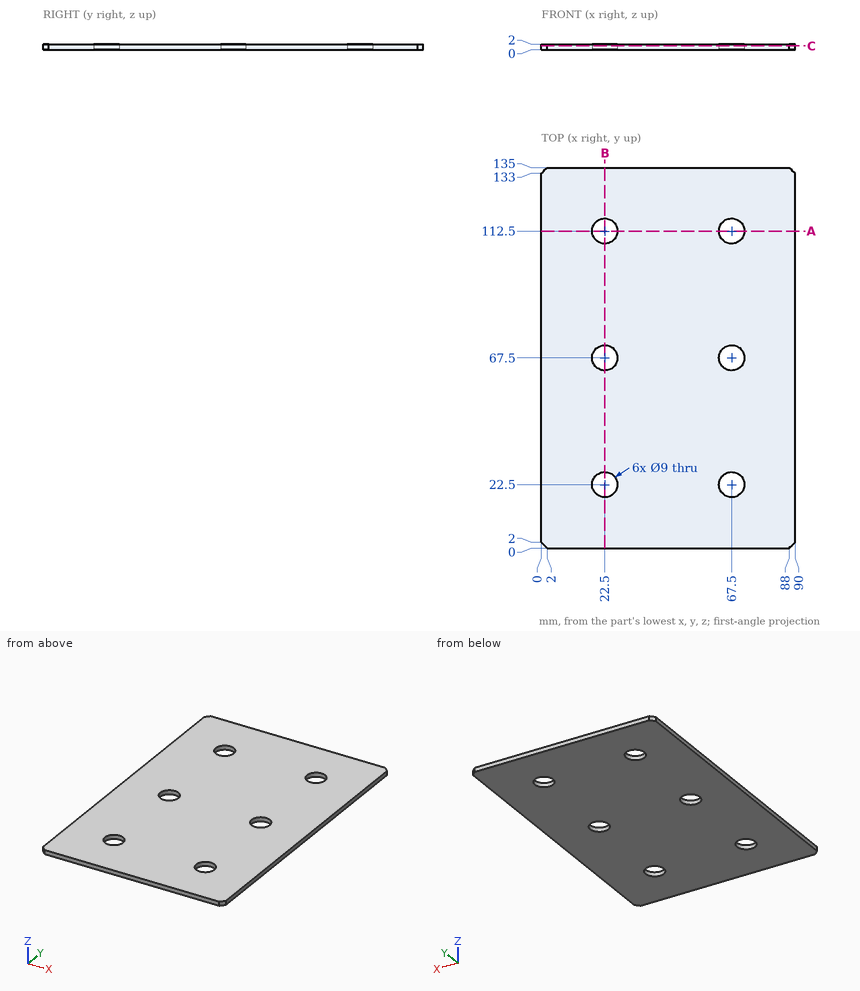
The drawing under review shows one solid part. Ordinate dimensions are in mm from its lowest x, y, z. Coordinates: 2 decimals unless noted, no trailing zeros. Order: outer loops, then holes, each group sorted by start corner. A loop starts at its lowest first (then second) coordinate and runs counter-clockwise, first axis right, second up. Notation, with made-up numbers: (-20, -12.75) -> (25, -12.75) arc R22 ccw to (25, 5.25) -> close; hole circle Ø4 at (5, 68). An arc over 180 degrees is marked (long way). Use CSV: the item, a comma, the result in double quotes. Start each with the question number.
Item 1: We need section A-A, the plane y = 112.5. Give the boundary of the cut face in (x, z), then the cut area to 3 significant figures.
Item 2: We need section C-C, the plane z = 1.3. Give the boundary of the cut face in (x, y), then the cut area to 3 significant figures.
Item 3: We need section B-B, the plane x = 22.5. Give the boundary of the cut face in (y, z), then the cut area to 3 significant figures.
Item 4: Wall thickness on probe 1 along Y at (x, z) = (67.5, 0.55); probe 2 along X at (y, z) = (21, 0.2); probe 3 along Y at (x, z) = (69, 1.5): over which ranges is each line inside the solid? List them lowest first.
Item 5: Insertion check: pin 1 (8 mm diameter, centred on x = 22.5, y = 112.5, fed in from +Z). The pin has a flat end and moves straight along its axis. Give the tip position at first contact, or say it passes through.
Derived:
1,outline,"(0, 0) -> (18, 0) -> (18, 2) -> (0, 2) -> close; (27, 0) -> (63, 0) -> (63, 2) -> (27, 2) -> close; (72, 0) -> (90, 0) -> (90, 2) -> (72, 2) -> close"
1,area,"144 mm^2"
2,outline,"(0, 2) -> (2, 0) -> (88, 0) -> (90, 2) -> (90, 133) -> (88, 135) -> (2, 135) -> (0, 133) -> close; hole circle Ø9 at (22.5, 22.5); hole circle Ø9 at (22.5, 67.5); hole circle Ø9 at (22.5, 112.5); hole circle Ø9 at (67.5, 22.5); hole circle Ø9 at (67.5, 67.5); hole circle Ø9 at (67.5, 112.5)"
2,area,"11,800 mm^2"
3,outline,"(0, 0) -> (18, 0) -> (18, 2) -> (0, 2) -> close; (27, 0) -> (63, 0) -> (63, 2) -> (27, 2) -> close; (72, 0) -> (108, 0) -> (108, 2) -> (72, 2) -> close; (117, 0) -> (135, 0) -> (135, 2) -> (117, 2) -> close"
3,area,"216 mm^2"
4,probe 1,"y = 0 to 18, 27 to 63, 72 to 108, 117 to 135"
4,probe 2,"x = 0 to 18.26, 26.74 to 63.26, 71.74 to 90"
4,probe 3,"y = 0 to 18.26, 26.74 to 63.26, 71.74 to 108.26, 116.74 to 135"
5,pin 1,"passes through"
